Study the drawing (mm; zero at the part's minimum x, y, z) and answer. A direction names the side the tool comes from. Coordinates: 2 decimals unless noted, no trailing zeros. Loops run counter-clockwise (first coordinate to the right, second up) from the corner with the lowest first, then second, coordinate; pieces in that order, holes last. Notation, with made-up numbers: (34.5, 45.25) - (79.5, 45.25) arc R8 cw to (79.5, 57.25) - close; hole circle Ø6 at (15, 44). An arc over 180 degrees is marked (long way). Put each result on its own line as item: value.
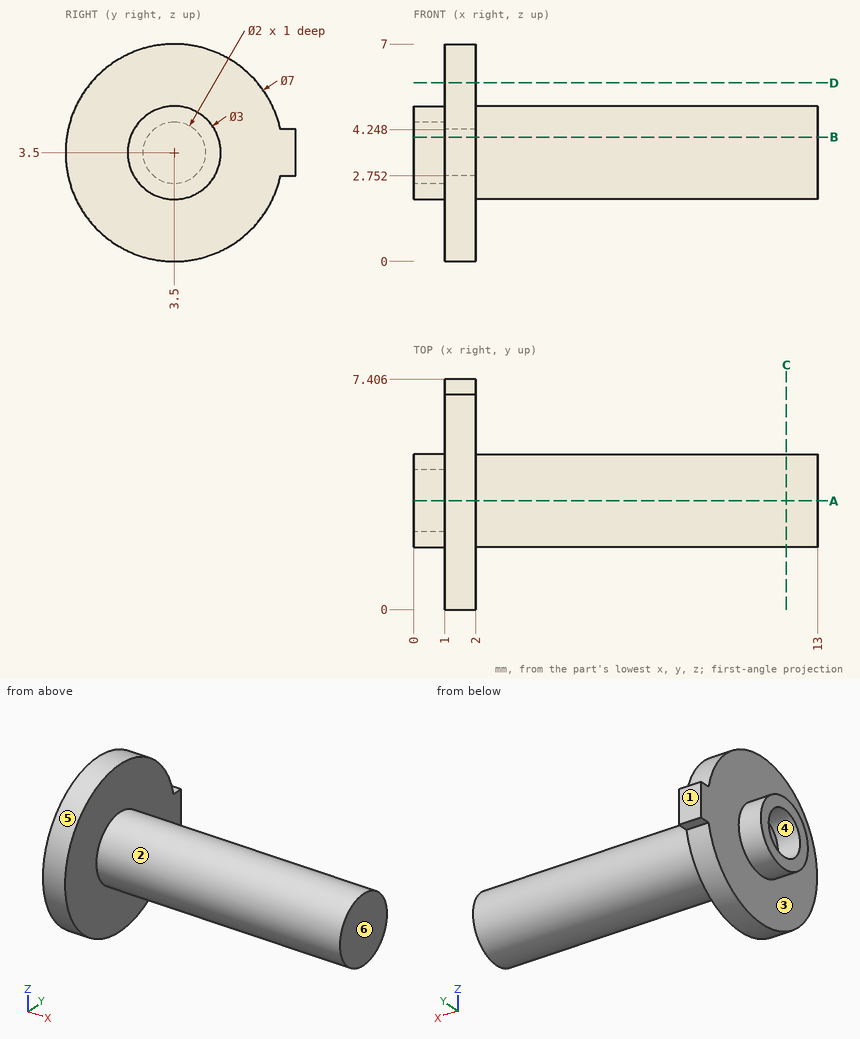
1) For a pull along Z with two mould halves and no side action, classify the marked faces 4, 5 and 6 as pulls with the +Z half, pulls with the -Z half, needs draft (parallel to the pull), parting line crosses it, or undercut.
Found:
face 4: undercut
face 5: parting line crosses it
face 6: needs draft
2) Straight lines are drawn through the part: L1, parallel to X at y = 4, z = 3; L2, parallel to X at y = 2.5, z = 4.75; L3, parallel to Y at x = 10.5, z = 2.25 (1 decimal). For each, find the intervals that lie inside material, in ascending order. Write a range as [from, to].
Found:
L1: x = [1, 13]
L2: x = [1, 2]
L3: y = [2.7, 4.3]
3) The part is cut by section A-A (y = 3.5). Give the vertices of the cut face in (x, z).
Found:
outline: (0, 2) - (1, 2) - (1, 0) - (2, 0) - (2, 2) - (13, 2) - (13, 5) - (2, 5) - (2, 7) - (1, 7) - (1, 5) - (0, 5) - (0, 4.5) - (1, 4.5) - (1, 2.5) - (0, 2.5) - close
4) The part is cut by section B-B (z = 4). Give the vertices of the cut face in (x, y) (1 decimal).
Found:
outline: (0, 2.1) - (1, 2.1) - (1, 0) - (2, 0) - (2, 2.1) - (13, 2.1) - (13, 4.9) - (2, 4.9) - (2, 7.4) - (1, 7.4) - (1, 4.9) - (0, 4.9) - (0, 4.4) - (1, 4.4) - (1, 2.6) - (0, 2.6) - close
5) Each of these flat-tipped pins is pushed along its axis until it touches: pin 1 (2 mm diameter, centred on y = 2.5, z = 2.5, fed in from -X); pin 2 (3 mm diameter, centred on x = 11.5, z = 3.5, fed in from -Y); pin 3 (1.5 mm diameter, centred on x = 5, y = 3, fed in from -Z). Where does it stop, or does it pass through?
Found:
pin 1: stops at x = 0
pin 2: stops at y = 2
pin 3: stops at z = 2
6) The part is cut by section C-C (x = 12). Give the vertices of the cut face in (y, z).
Found:
outline: circle Ø3 at (3.5, 3.5)
7) For the marked faces 1, 2 and 3, determine the directions among +Z, -Z, +X, -X, +Y, -Y from which every point of the face is accessible in a straight line to the end or side of a thin tool.
Found:
face 1: +Z, -Z, +X, -X, +Y
face 2: +X
face 3: -X
8) The part is cut by section D-D (z = 5.75). Give the vertices of the cut face in (x, y).
Found:
outline: (1, 0.82) - (2, 0.82) - (2, 6.18) - (1, 6.18) - close
